Solid Edge part; units mm, degrees
sketch "Sketch1" plane through (0, 0, 0) normal (0, -1, 0) x (1, 0, 0)
  line L0 (60.007, 20) -> (60.007, 0)
  line L1 (60.007, 0) -> (0, 0)
  line L2 (0, 0) -> (0, 20)
  line L3 (0, 20) -> (60.007, 20)
extrude "Protrusion1" add sketch "Sketch1" along normal blind 50
sketch "Sketch2" plane through (60.007, -20, 10) normal (1, 0, 0) x (0, 1, 0)
  circle A0 centre (-5, 10) radius 15
extrude "ExtrudedCutout_1" cut sketch "Sketch2" against normal blind 100
sketch "Sketch3" plane through (30.0035, -45, 20) normal (0, 0, 1) x (-1, 0, 0)
  circle A0 centre (20.0035, 0) radius 2.5
extrude "Cutout1" cut sketch "Sketch3" against normal blind 100
mirror "Mirror1" about plane through (30.003, -25, 10) normal (-1, 0, 0) of "Cutout1"
mirror "Mirror2" about plane through (30.0035, -25, 10) normal (0, 1, 0) of "Cutout1", "Mirror1"
Model file for the job. Use its own axes, mm. Coordinates: 2 decimals unless noted, no trailing zeros. Write each loop counter-clockwise with the first axis right and the second up, starting at its lowest first coordinate (ties: lowest second). Pieces come first, ordered by that corner, then holes. Notation, with made-up numbers: (53, -2) -> (82, -2) arc R11 ccw to (82, 11) -> close; hole circle Ø7 at (9, 60.25). An arc over 180 degrees is marked (long way). One line per item, written item: value. Start each with the question number.
1) Pull direction Y, two halves, no side cores. Call faces 1 (the face through (30, -50, 10)), 2 (the face through (10.54, -42.56, 10.14)), 3 (the face through (30, -25, 5)), 4 (the face through (30, -5, 20)): +Y half, -Y half, draft (parallel to the pull), parting line (faces both ways), or undercut.
2) Slice it at A-A on z = 16.5. Write the cut outline in (x, y), then the cut area to 3 significant figures.
3) Flat gauge pins, fed straight in: pin 1 Ø4.5 at (x, y) = (50.006, -5) entering from +Z; pin 2 Ø8 at (x, y) = (23, -33.5) entering from +Z. Where does each tip first touch, or does it go through?
4) Probe probe 1 along X at (y, z) = (-45, 10.75); probe 2 along X at (y, z) = (-47, 11.75); probe 3 along Y at (x, z) = (10, 13.5). List the from-to ranges inside material, lowest first.
5) Slice it at D-D on z = 3.5. Write the cut outline in (x, y), then the cut area to 3 significant figures.
6) Slice it at B-B on x = 11.5. Write the cut outline in (y, z).
7) Slice it at C-C on y = -5. Write the cut outline in (x, z), then the cut area to 3 significant figures.
Answers follow:
1. face 1: -Y half
1. face 2: undercut
1. face 3: undercut
1. face 4: draft
2. outline: (0, -50) -> (60.01, -50) -> (60.01, -39.59) -> (0, -39.59) -> close; (0, -10.41) -> (60.01, -10.41) -> (60.01, 0) -> (0, 0) -> close; hole circle Ø5 at (10, -45); hole circle Ø5 at (10, -5); hole circle Ø5 at (50.01, -45); hole circle Ø5 at (50.01, -5)
2. area: 1,170 mm2
3. pin 1: through
3. pin 2: z = 11.71
4. probe 1: 0 to 7.5, 12.5 to 47.51, 52.51 to 60.01
4. probe 2: 0 to 8.5, 11.5 to 48.51, 51.51 to 60.01
4. probe 3: -50 to -47.5, -42.5 to -38.52, -11.48 to -7.5, -2.5 to 0
5. outline: (0, -50) -> (60.01, -50) -> (60.01, 0) -> (0, 0) -> close; hole circle Ø5 at (10, -45); hole circle Ø5 at (10, -5); hole circle Ø5 at (50.01, -45); hole circle Ø5 at (50.01, -5)
5. area: 2,920 mm2
6. outline: (-50, 0) -> (-47, 0) -> (-47, 20) -> (-50, 20) -> close; (-43, 0) -> (-7, 0) -> (-7, 20) -> (-10, 20) arc R15 cw to (-40, 20) -> (-43, 20) -> close; (-3, 0) -> (0, 0) -> (0, 20) -> (-3, 20) -> close
7. outline: (0, 0) -> (7.5, 0) -> (7.5, 20) -> (0, 20) -> close; (12.5, 0) -> (47.51, 0) -> (47.51, 20) -> (12.5, 20) -> close; (52.51, 0) -> (60.01, 0) -> (60.01, 20) -> (52.51, 20) -> close
7. area: 1,000 mm2
